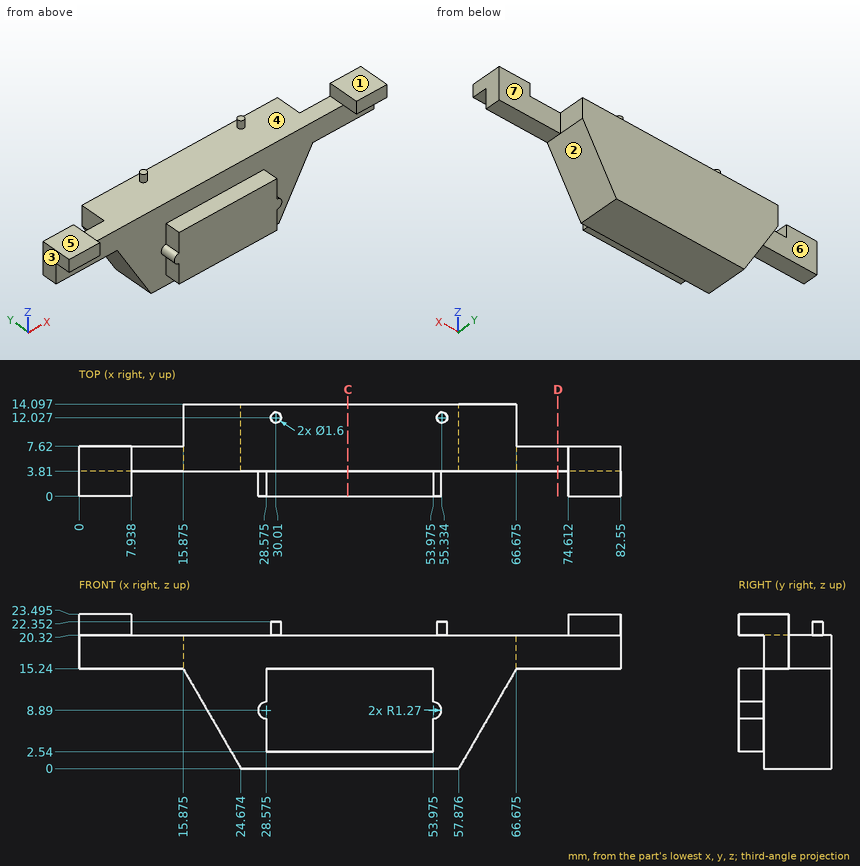
Job drawing, mm, ordinate dimensions from the low corner. One solid piece. A direction names the side the tool comes from. Give positions to 0.01 mm unless a question says otherwise; leave off trailing zeros. Loops run counter-clockwise (first coordinate to the right, second up) from the corner with the lowest first, then second, coordinate; pieces in that order, holes last.
Item 1: Which spindle directions (+Z, -Z, +X, -X, +Y, -Y) get a long thin tool onto all of the face, cutting with end or side? Do the marked faces 5, 6 and 7. Say none if no direction does.
Answers follow:
face 5: +Z, +X, -X, +Y, -Y
face 6: +Z, -Z, -X, +Y
face 7: +Z, -Z, +X, +Y
Item 2: Slice it at C-C, the plane x = 41. List the corners of the cut face in (y, z).
Answers follow:
outline: (0, 2.54) - (3.81, 2.54) - (3.81, 0) - (14.1, 0) - (14.1, 20.32) - (3.81, 20.32) - (3.81, 15.24) - (0, 15.24) - close
Item 3: Flat gauge pins, fed straight in: pin 1 (2 mm diameter, centred on x = 29.5, y = 4.5, fed in from +Z); pin 2 (4 mm diameter, centred on y = 10, z = 18, fed in from +X) (1 decimal); pin 3 (1.1 mm diameter, centred on y = 2.5, z = 5.5, fed in from -X) (1 decimal); pin 4 (1 mm diameter, centred on y = 2.5, z = 19, fed in from -X). Where does each tip first touch, or does it go through?
Answers follow:
pin 1: stops at z = 20.32
pin 2: stops at x = 66.7
pin 3: stops at x = 28.6
pin 4: passes through
Item 4: Drill centre lines: line 1 (Y direction, x = 32.5, z = 15.75); line 2 (Z direction, x = 27.5, y = 11); line 3 (Z direction, x = 7, y = 6.25) (1 decimal). Where is each one in solid material? Low to high.
Answers follow:
line 1: y = 3.81 to 14.1
line 2: z = 0 to 20.32
line 3: z = 15.2 to 23.5
Item 5: Slice it at D-D, the plane x = 73. List the corners of the cut face in (y, z).
Answers follow:
outline: (3.81, 15.24) - (7.62, 15.24) - (7.62, 20.32) - (3.81, 20.32) - close
Item 6: Pull direction X, two halves, no side cores. Call the marked faces 1, 2, 3 and 4: released by +X, released by -X, zero draft, split by the parting line, or undercut.
Answers follow:
face 1: zero draft
face 2: released by +X
face 3: released by -X
face 4: undercut
